from build123d import *

# Parameters (mm, degrees)
F1_DEPTH      = 14
F2_R          = 2.75
F3_DEPTH      = 32.801
F4_SIZE       = 1
F5_R          = 0.6
F6_SIZE       = 0.6
F7_R          = 1.9
F8_DEPTH      = 20.501
F8_DEPTH_BACK = 21.501
F9_R          = 2.25
F10_DEPTH     = 9.5
F11_R         = 3
F12_DEPTH     = 4


with BuildPart() as f1:
    # F0 (on Front) → F1 (new body)
    with BuildSketch(Plane.XZ):
        with BuildLine():
            Line((-21, 0), (0, 0))
            Line((0, 0), (21, 0))
            Line((21, 0), (21, 6))
            Line((21, 6), (9, 6))
            Line((9, 6), (9, 32.8))
            Line((9, 32.8), (0.5, 32.8))
            Line((0.5, 32.8), (0.5, 24.9749371855))
            ThreePointArc((0.5, 24.9749371855), (0, 15), (-0.5, 24.9749371855))
            Line((-0.5, 24.9749371855), (-0.5, 32.8))
            Line((-0.5, 32.8), (-9, 32.8))
            Line((-9, 32.8), (-9, 6))
            Line((-9, 6), (-21, 6))
            Line((-21, 6), (-21, 0))
        make_face()
    extrude(amount=F1_DEPTH)

    # F2 (on face) → F3 (cut, through all)
    with BuildSketch(Plane(origin=(0, 0, 0), x_dir=(1, 0, 0), z_dir=(0, 0, -1))):
        with Locations((-16, 7)):
            Circle(F2_R)
        with Locations((16, 7)):
            Circle(F2_R)
    extrude(amount=-F3_DEPTH, mode=Mode.SUBTRACT)

    # F4
    f4_edges = [f1.edges().sort_by_distance(p)[0] for p in [
        (0, -14, 15),
        (0, 0, 15),
    ]]
    chamfer(f4_edges, length=F4_SIZE)

    # F5
    f5_edges = [f1.edges().sort_by_distance(p)[0] for p in [
        (9, -7, 6),
        (-9, -7, 6),
    ]]
    fillet(f5_edges, radius=F5_R)

    # F6
    f6_edges = [f1.edges().sort_by_distance(p)[0] for p in [
        (13.25, -7, 6),
        (-18.75, -7, 6),
    ]]
    chamfer(f6_edges, length=F6_SIZE)

    # F7 (on face) → F8 (cut, two sides)
    with BuildSketch(Plane.YZ.offset(-0.5)) as f8_sk:
        with Locations((-7, 28.8874685928)):
            Circle(F7_R)
    extrude(amount=-F8_DEPTH, mode=Mode.SUBTRACT)
    extrude(f8_sk.sketch, amount=F8_DEPTH_BACK, mode=Mode.SUBTRACT)

    # F9 (on face) → F10 (cut, through all)
    with BuildSketch(Plane.YZ.offset(9)):
        with Locations((-7, 28.8874685928)):
            Circle(F9_R)
    extrude(amount=-F10_DEPTH, mode=Mode.SUBTRACT)

    # F11 (on face) → F12 (cut)
    with BuildSketch(Plane.YZ.offset(9)):
        with Locations((-7, 28.8874685928)):
            Circle(F11_R)
    extrude(amount=-F12_DEPTH, mode=Mode.SUBTRACT)


solid = f1.part
Verification items for the finished model (mm, model axes). A direction names the side the tool comes from. Give positions to 0.01 mm unless a question says otherwise; leave off trailing zeros. Order: outer loops, then holes, each group sorted by start corner. A loop starts at its lowest first (then second) coordinate and runs counter-clockwise, first axis right, second up. Notation, with made-up numbers: M 20,13.5 L 61,13.5 A5 cw 61,18.5 Z; hole C 4.25,-33.75 d11. An arc over 180 degrees is marked long. Use one line per item in the form item = value. Start each with the question number.
Q1. Section check C-C (z = 2.5). Enter the section's corners in (x, y), then the cut area to 3 significant figures.
Q2. Section check D-D (x = 0). Enter the section's corners in (y, z), then the cut area to 3 significant figures.
Q3. Access from +Z, -Z, +X, -X, +Y, -Y to the whole of each face (thin tool, end or side, straight path). Record for faces 4 (the flat face through (12.8, -8.5, 6)), 5 (the cylindrical face through (2.78, -7.29, 31.12)), 6 (the flat face through (-9, -7, 20)), 7 (the flat face through (0, -7, 0)), 8 (the flat face through (-0.5, -5, 31)).
Q4. Go/stop test with flat-tipped pins: pin 1 Ø3 at (y, z) = (-4, 21) entering from -X; pin 2 Ø13 at (x, z) = (0, 20) entering from +Y; pin 3 Ø8 at (y, z) = (-7, 28.89) entering from +X; pin 4 Ø3.5 at (x, y) = (16, -7) entering from +Z. Record where each tip stops, or that it passes through.
Q5. Scan lines: line 1 along X through (y, z) = (-7, 3.3); line 2 along Y through (x, z) = (-1.5, 29); line 3 along X through (y, z) = (-4.5, 2). Record each from-to range of solid material in increasing order. Write a range as [from, to].
Q6. Mould release check, pull along Y, two halves, no side actions. Record for faces 1 (the cylindrical face through (-4.69, -7.412, 27.033)), 2 (the conical face through (0.221, -0.84, 14.845)), 3 (the flat face through (5, -7, 32.8)): +Y half, -Y half, draft (parallel to the pull), parting line (faces both ways), or undercut.
Q7. Section check A-A (x = 16). Enter the section's corners in (y, z).
Q8. Section check B-B (z = 20). Enter the section's corners in (x, y), then the cut area to 3 significant figures.
Evaluation:
q1.outline = M -21,-14 L 21,-14 L 21,0 L -21,0 Z; hole C -16,-7 d5.5; hole C 16,-7 d5.5
q1.area = 540 mm2
q2.outline = M -14,0 L 0,0 L 0,14 L -1,15 L -13,15 L -14,14 Z
q2.area = 209 mm2
q3.face_4 = +Z, +X, +Y, -Y
q3.face_5 = +X
q3.face_6 = +Z, -X, +Y, -Y
q3.face_7 = -Z, +X, -X, +Y, -Y
q3.face_8 = +Z, +Y, -Y
q4.pin_1 = -9
q4.pin_2 = 0
q4.pin_3 = 9
q4.pin_4 = through
q5.line_1 = [-21, -18.75], [-13.25, 13.25], [18.75, 21]
q5.line_2 = [-14, -8.9], [-5.1, 0]
q5.line_3 = [-21, -17.15], [-14.85, 14.85], [17.15, 21]
q6.face_1 = undercut
q6.face_2 = +Y half
q6.face_3 = draft
q7.outline = M -14,0 L -9.75,0 L -9.75,5.4 L -10.35,6 L -14,6 Z; M -4.25,0 L 0,0 L 0,6 L -3.65,6 L -4.25,5.4 Z
q8.outline = M -9,-14 L -6,-14 L -5,-13 L -5,-1 L -6,0 L -9,0 Z; M 5,-13 L 6,-14 L 9,-14 L 9,0 L 6,0 L 5,-1 Z
q8.area = 110 mm2
